Geometry check sheet. Reference: the model listing, model coordinates, mm. A direction names the side the tool comes from. Coordinates: 2 decimals unless noted, no trailing zeros. Order: outer loops, then holes, each group sorted by start corner. A loop starts at its lowest first (then second) coordinate and runs counter-clockwise, first axis right, second up. Notation, with made-up numbers: (48, 46.25) - (73, 46.25) arc R15 cw to (73, 55.25) - close; hole circle Ø6 at (52.25, 55.25). An arc over 180 degrees is marked (long way). Return JSON: item names as keys, results as strings. Group by question number.
Item 1: Tool access check on faces 1 (the cylindrical face through (-1.73, -7.81, -0.44)), 2 (the flat face through (0, -13, -28.05)). Record the directions out of +Z, -Z, +X, -X, +Y, -Y that give a thin tool (end or side, any length) a straight path to the whole face; none if there is none.
Item 2: Gauge pin test, flat ends, axial feed: pin 1 (8 mm diameter, centred on x = -8, z = -23.5, fed in from -Y); pin 2 (8 mm diameter, centred on y = -22.5, z = 9.5, fed in from +X); pin 3 (3 mm diameter, centred on y = 21, z = 23.5, fed in from +X). Record the tip position at first contact, or that the pin passes through.
Item 3: Section check D-D on x = -10.5. Enter the section's corners in (y, z), then the cut area to 3 significant figures.
Item 4: Section check A-A on y = 0. Enter the section's corners in (x, z).
Item 5: Scan lines: probe 1 along Y at (x, z) = (0, -9); probe 2 along X at (y, z) = (1, 2); probe 3 along Y at (x, z) = (-3, 11.5). Record each from-to range of solid material in increasing order.
Item 6: Section check C-C on z = 14.5. Enter the section's corners in (x, y).
Item 7: Draft check along Z on faces 3 (the cylindrical face through (18.28, 28.67, 0.44)), 4 (the cylindrical face through (-1.5, 11.4, -0.4)), 5 (the flat face through (7, -7, -31.55)), 6 (the cylindrical face through (-24.204, -18.559, 0.393)). Enter one of: pulls with the +Z half, pulls with the -Z half, needs draft (parallel to the pull), parting line crosses it, or undercut.
from build123d import *

# Parameters (mm, degrees)
SKETCH1_R           = 34
SKETCH1_R_2         = 8
BOSS_EXTRUDE1_DEPTH = 31.55
SHELL1_T            = 3.5


with BuildPart() as part:
    # Sketch1 → Boss-Extrude1 (new, symmetric)
    with BuildSketch(Plane.XY):
        Circle(SKETCH1_R)
        Circle(SKETCH1_R_2, mode=Mode.SUBTRACT)
    extrude(amount=BOSS_EXTRUDE1_DEPTH, both=True)

    # Shell1 (no face opened: a closed hollow body)
    add(offset(amount=-SHELL1_T, mode=Mode.PRIVATE), mode=Mode.SUBTRACT)


solid = part.part
Computed:
{
 "1": {"face 1": "+Z, -Z", "face 2": "none"},
 "2": {"pin 1": "stops at y = -33.76", "pin 2": "stops at x = 28.53", "pin 3": "stops at x = 27.85"},
 "3": {"outline": "(-32.34, -31.55) - (32.34, -31.55) - (32.34, 31.55) - (-32.34, 31.55) - close; hole (-28.64, -28.05) - (-4.69, -28.05) - (-4.69, 28.05) - (-28.64, 28.05) - close; hole (4.69, -28.05) - (28.64, -28.05) - (28.64, 28.05) - (4.69, 28.05) - close", "area": "1,390 mm²"},
 "4": {"outline": "(-34, -31.55) - (-8, -31.55) - (-8, 31.55) - (-34, 31.55) - close; (8, -31.55) - (34, -31.55) - (34, 31.55) - (8, 31.55) - close; hole (-30.5, -28.05) - (-11.5, -28.05) - (-11.5, 28.05) - (-30.5, 28.05) - close; hole (11.5, -28.05) - (30.5, -28.05) - (30.5, 28.05) - (11.5, 28.05) - close"},
 "5": {"probe 1": "y = -34 to -30.5, -11.5 to -8, 8 to 11.5, 30.5 to 34", "probe 2": "x = -33.99 to -30.48, -11.46 to -7.94, 7.94 to 11.46, 30.48 to 33.99", "probe 3": "y = -33.87 to -30.35, -11.1 to -7.42, 7.42 to 11.1, 30.35 to 33.87"},
 "6": {"outline": "circle Ø68 at (0, 0); circle Ø23 at (0, 0); hole circle Ø61 at (0, 0); hole circle Ø16 at (0, 0)"},
 "7": {"face 3": "needs draft", "face 4": "undercut", "face 5": "pulls with the -Z half", "face 6": "undercut"}
}
